The listing builds one solid part. Answer for the finished solid, in the listing's coordinates (mm). Face numbers are marked on the shaded views. A direction names the side the tool comes from. Give positions to 0.01 mm unless a question says otherwise; leave off trailing zeros. Loops run counter-clockwise (first coordinate to the right, second up) from the corner with the lowest first, then second, coordinate; pieces in that order, holes last. Notation, with made-up numbers: (48.25, 6) - (79.25, 6) arc R11 ccw to (79.25, 19) - close; hole circle Ø6 at (4, 85). An arc over 180 degrees is marked (long way). Write item = value, one per line. Start each with the question number.
1) Consider probe 1 along X at (y, z) = (14.5, -24); probe 2 along Y at (x, z) = (-26.35, -4); probe 3 along Z at (x, y) = (26.55, 5). Determine where each line is inside the solid, lowest interval first.
2) The part is cut by section A-A on y = 5. Write down the section's boundary in (x, z).
3) The part is cut by section D-D on z = -19.5. Write down the section's boundary in (x, y).
4) Flat-ended cylindrical pins translate along their axes: P1, Ø12, axis at y = 8.5, z = -34.5, coming from the -X side; P2, Ø5, axis at x = -30, z = -42.5, coming from the +Y side; P3, Ø5, axis at x = 0.5, y = 6, coming from the -Z side. Find the tip coordinate at first contact, or state that the pin passes through.
5) The part is cut by section C-C on x = 9.5. Write down the section's boundary in (y, z), plus the area to 3 significant figures.
6) The mould has two halves that part along Z. Classify the marked faces 4, 5 and 6: +Z half, -Z half, draft (parallel to the pull), parting line (faces both ways), or undercut.
7) The part is cut by section B-B on z = -4. Write down the section's boundary in (x, y), plus the area to 3 significant figures.
8) Which of the six approach directions +Z, -Z, +X, -X, +Y, -Y give full straight-line access (tool end or side, diameter ignored) to the marked faces 1, 2 and 3?
from build123d import *

# Parameters (mm, degrees)
CROQUIS1_R              = 2.1
SALIENTE_EXTRUIR1_DEPTH = 27
CROQUIS2_W              = 50
CROQUIS2_H              = 35.661242199
CORTAR_EXTRUIR1_DEPTH   = 20
CROQUIS3_W              = 94
CROQUIS3_H              = 22
SALIENTE_EXTRUIR2_DEPTH = 2
CROQUIS4_W              = 94
CROQUIS4_H              = 57.661242199
SALIENTE_EXTRUIR3_DEPTH = 2


with BuildPart() as part:
    # Croquis1 → Saliente-Extruir1 (new body, symmetric)
    with BuildSketch(Plane(origin=(0, 0, 0), x_dir=(0, 0, -1), z_dir=(1, 0, 0))):
        Polygon((0, 0), (0, 20), (11.90751736, 20), (37.661242199, 10), (37.661242199, 0), align=None)
        with Locations((4, 5)):
            Circle(CROQUIS1_R, mode=Mode.SUBTRACT)
    extrude(amount=SALIENTE_EXTRUIR1_DEPTH, both=True)

    # Croquis2 → Cortar-Extruir1 (cut)
    with BuildSketch(Plane(origin=(0, 20, 0), x_dir=(1, 0, 0), z_dir=(0, 1, 0))):
        with Locations((0, 17.8306211)):
            Rectangle(CROQUIS2_W, CROQUIS2_H)
    extrude(amount=-CORTAR_EXTRUIR1_DEPTH, mode=Mode.SUBTRACT)

    # Croquis3 → Saliente-Extruir2 (add)
    with BuildSketch(Plane.XY):
        with Locations((0, 9)):
            Rectangle(CROQUIS3_W, CROQUIS3_H)
    extrude(amount=SALIENTE_EXTRUIR2_DEPTH)

    # Croquis4 → Saliente-Extruir3 (add)
    with BuildSketch(Plane.XZ):
        with Locations((0, -28.8306211)):
            Rectangle(CROQUIS4_W, CROQUIS4_H)
    extrude(amount=SALIENTE_EXTRUIR3_DEPTH)


solid = part.part
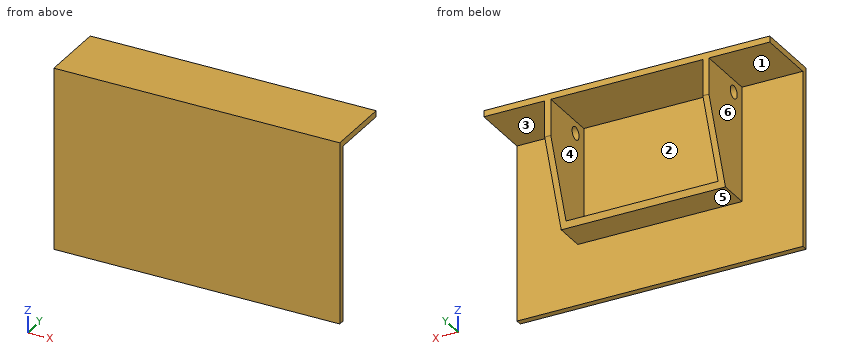
Answer below:
q1.probe_1 = -27 to -25, 25 to 27
q1.probe_2 = -2 to 2.9, 7.1 to 20
q1.probe_3 = -37.66 to -6.1, -1.9 to 2
q2.outline = (-47, 0) - (-27, 0) - (-27, -1.9) - (-25, -1.9) - (-25, 0) - (25, 0) - (25, -1.9) - (27, -1.9) - (27, 0) - (47, 0) - (47, 2) - (-47, 2) - close; (-27, -37.66) - (27, -37.66) - (27, -6.1) - (25, -6.1) - (25, -35.66) - (-25, -35.66) - (-25, -6.1) - (-27, -6.1) - close
q3.outline = (-47, -2) - (47, -2) - (47, 0) - (27, 0) - (27, 17.05) - (25, 17.05) - (25, 0) - (-25, 0) - (-25, 17.05) - (-27, 17.05) - (-27, 0) - (-47, 0) - close
q4.P1 = -27
q4.P2 = 0
q4.P3 = -37.66
q5.outline = (-2, -57.66) - (0, -57.66) - (0, -37.66) - (10, -37.66) - (10.78, -35.66) - (0, -35.66) - (0, 0) - (20, 0) - (20, 2) - (-2, 2) - close
q5.area = 180 mm2
q6.face_4 = undercut
q6.face_5 = -Z half
q6.face_6 = draft
q7.outline = (-47, -2) - (47, -2) - (47, 0) - (27, 0) - (27, 2.9) - (25, 2.9) - (25, 0) - (-25, 0) - (-25, 2.9) - (-27, 2.9) - (-27, 0) - (-47, 0) - close; (-27, 7.1) - (-25, 7.1) - (-25, 20) - (-27, 20) - close; (25, 7.1) - (27, 7.1) - (27, 20) - (25, 20) - close
q7.area = 251 mm2
q8.face_1 = -Z, -X, +Y
q8.face_2 = +Y
q8.face_3 = -Z, +X, +Y
